```python
from build123d import *

# Parameters (mm, degrees)
SKETCH008_W     = 14
SKETCH008_H     = 42
PAD002_DEPTH    = 13
SKETCH010_W     = 13
SKETCH010_H     = 40
POCKET006_DEPTH = 13.001
SKETCH011_W     = 10
SKETCH011_H     = 1
PAD004_DEPTH    = 10
SKETCH012_R     = 0.75
PAD005_DEPTH    = 3


with BuildPart() as sensor_case:
    # Sketch008 → Pad002 (new body)
    with BuildSketch(Plane.XY):
        with Locations((7, 21)):
            Rectangle(SKETCH008_W, SKETCH008_H)
    extrude(amount=PAD002_DEPTH)

    # Sketch010 (on Face6 of Pad002) → Pocket006 (cut, through all)
    with BuildSketch(Plane.XY.offset(13)):
        with Locations((6.5, 21)):
            Rectangle(SKETCH010_W, SKETCH010_H)
    extrude(amount=-POCKET006_DEPTH, mode=Mode.SUBTRACT)

    # Sketch011 → Pad004 (join)
    with BuildSketch(Plane(origin=(0, 1, 0), x_dir=(-1, 0, 0), z_dir=(0, 1, 0))):
        with Locations((-8, 0.5)):
            Rectangle(SKETCH011_W, SKETCH011_H)
    extrude(amount=PAD004_DEPTH)

    # Sketch012 (on Face13 of Pad004) → Pad005 (join)
    with BuildSketch(Plane.XY.offset(1)):
        with Locations((9.5, 8)):
            Circle(SKETCH012_R)
    extrude(amount=PAD005_DEPTH)


with BuildPart() as sensor_case_1:
    # Body001 placement: moved
    add(sensor_case.part.moved(Location((0, 0, 14))))


with BuildPart() as mirrored_sensor_case:
    # Part__Mirroring001: instance of Sensor Case
    add(sensor_case_1.part.mirror(Plane(origin=(0, 0, 0), x_dir=(0, -1, 0), z_dir=(1, 0, 0))))


solid = mirrored_sensor_case.part
```
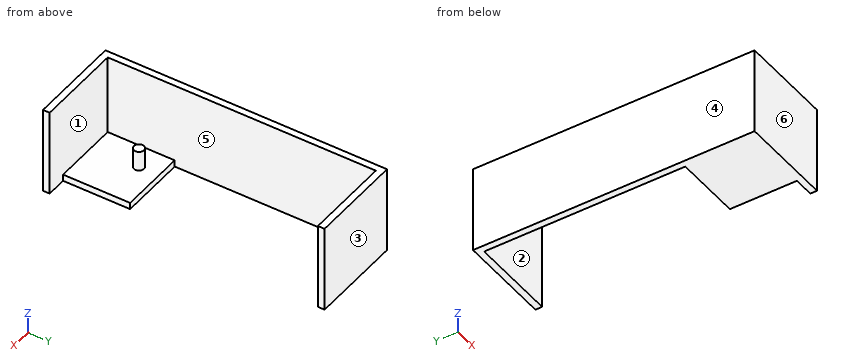
Check sheet for the modelled part. Datum: model origin and axes. Units: mm. Face numbers are marked on the shaded views. A direction names the side the tool comes from. Round coordinates to 2 decimals unless told otherwise and drop trailing zeros. Order: outer loops, then holes, each group sorted by start corner. A loop starts at its lowest first (then second) coordinate and runs counter-clockwise, first axis right, second up.
1) Section check B-B (x = -5.5). Record the boundary of the cut face in (y, z), and give its area (3 significant figures).
2) Section check C-C (z = 18.5). Record the boundary of the cut face in (x, y).
3) Mould release check, pull along Y, two halves, no side actions. Record for the marked faces 4, 5 and 6: +Y half, -Y half, draft (parallel to the pull), parting line (faces both ways), or undercut.
4) Scan lines: line 1 (Y direction, x = -6.75, z = 23.25); line 2 (Z direction, x = -7.5, y = 8); line 3 (X direction, y = 15, z = 25.5). Record each from-to range of solid material in increasing order.
5) Tool access check on the marked faces 1, 2 and 3. Record the directions out of +Z, -Z, +X, -X, +Y, -Y that give a thin tool (end or side, any length) a straight path to the whole face; none if there is none.
6) Section check A-A (z = 16.25). Record the boundary of the cut face in (x, y).
7) Go/stop test with flat-tipped pins: pin 1 Ø1 at (y, z) = (25, 24.5) entering from +X; pin 2 Ø8 at (x, y) = (-4, 16) entering from -Z; pin 3 Ø0.8 at (y, z) = (4.5, 14.5) entering from +X. Record where each tip stops, or that it passes through.
8) Section check D-D (y = 10). Record the boundary of the cut face in (x, z).
Result:
1. outline: (0, 14) - (11, 14) - (11, 15) - (1, 15) - (1, 27) - (0, 27) - close; (41, 14) - (42, 14) - (42, 27) - (41, 27) - close
1. area: 36.0 mm2
2. outline: (-14, 0) - (0, 0) - (0, 1) - (-13, 1) - (-13, 41) - (0, 41) - (0, 42) - (-14, 42) - close
3. face 4: draft
3. face 5: undercut
3. face 6: -Y half
4. line 1: y = 0 to 1, 41 to 42
4. line 2: z = 14 to 15
4. line 3: x = -14 to -13
5. face 1: +Z, +X
5. face 2: +Z, -Z, +X
5. face 3: +Z, -Z, +X, -X, +Y
6. outline: (-14, 0) - (0, 0) - (0, 1) - (-13, 1) - (-13, 41) - (0, 41) - (0, 42) - (-14, 42) - close; circle Ø1.5 at (-9.5, 8)
7. pin 1: stops at x = -13
7. pin 2: passes through
7. pin 3: stops at x = -3
8. outline: (-14, 14) - (-3, 14) - (-3, 15) - (-13, 15) - (-13, 27) - (-14, 27) - close
